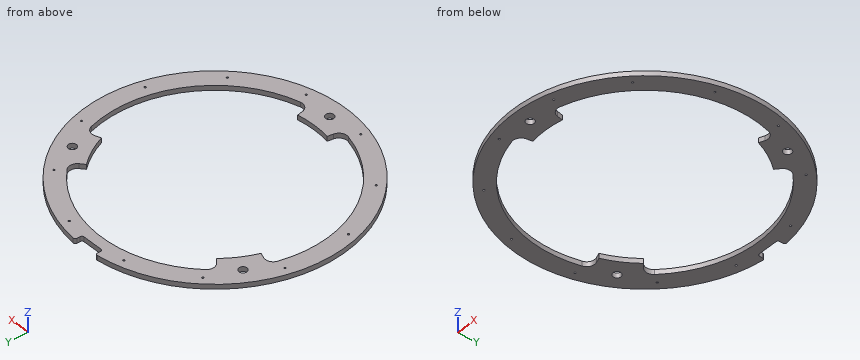
from build123d import *

# Parameters (mm, degrees)
SKETCH2_R                                      = 330
SKETCH2_R_2                                    = 250
BOSS_EXTRUDE1_DEPTH                            = 12
CUT_EXTRUDE1_DEPTH                             = 12
SKETCH4_R                                      = 10
CUT_EXTRUDE2_DEPTH                             = 12
SKETCH5_W                                      = 60
SKETCH5_H                                      = 60
CUT_EXTRUDE3_DEPTH                             = 12
FILLET1_R                                      = 5
CSK_FOR_M4_FLAT_HEAD_MACHINE_SCREW_D           = 4.5
CSK_FOR_M4_FLAT_HEAD_MACHINE_SCREW_CSINK_D     = 9.4
CSK_FOR_M4_FLAT_HEAD_MACHINE_SCREW_CSINK_ANGLE = 90


with BuildPart() as part:
    # Sketch2 → Boss-Extrude1 (new body)
    with BuildSketch(Plane.XY):
        Circle(SKETCH2_R)
        Circle(SKETCH2_R_2, mode=Mode.SUBTRACT)
    extrude(amount=BOSS_EXTRUDE1_DEPTH)

    # Sketch3 → Cut-Extrude1 (cut)
    with BuildSketch(Plane.XY.offset(12)):
        with BuildLine():
            Line((191.51111078, 160.696902422), (202.422805046, 169.852901056))
            ThreePointArc((202.422805046, 169.852901056), (209.542560602, 184.184300077), (203.874000238, 199.14917029))
            ThreePointArc((203.874000238, 199.14917029), (0, 285), (-203.874000238, 199.14917029))
            ThreePointArc((-203.874000238, 199.14917029), (-209.542560602, 184.184300077), (-202.422805046, 169.852901056))
            Line((-202.422805046, 169.852901056), (-191.51111078, 160.696902422))
            ThreePointArc((-191.51111078, 160.696902422), (0, 250), (191.51111078, 160.696902422))
        make_face()
        with BuildLine():
            Line((43.412044417, -246.201938253), (45.885524698, -260.229742003))
            ThreePointArc((45.885524698, -260.229742003), (54.737002544, -273.561330694), (70.531240495, -276.134648522))
            ThreePointArc((70.531240495, -276.134648522), (246.817240079, -142.5), (274.405240732, 76.985478232))
            ThreePointArc((274.405240732, 76.985478232), (264.279563146, 89.377030617), (248.308329744, 90.376840947))
            Line((248.308329744, 90.376840947), (234.923155196, 85.505035831))
            ThreePointArc((234.923155196, 85.505035831), (216.506350946, -125), (43.412044417, -246.201938253))
        make_face()
        with BuildLine():
            Line((-234.923155196, 85.505035831), (-248.308329744, 90.376840947))
            ThreePointArc((-248.308329744, 90.376840947), (-264.279563146, 89.377030617), (-274.405240732, 76.985478232))
            ThreePointArc((-274.405240732, 76.985478232), (-246.817240079, -142.5), (-70.531240495, -276.134648522))
            ThreePointArc((-70.531240495, -276.134648522), (-54.737002544, -273.561330694), (-45.885524698, -260.229742003))
            Line((-45.885524698, -260.229742003), (-43.412044417, -246.201938253))
            ThreePointArc((-43.412044417, -246.201938253), (-216.506350946, -125), (-234.923155196, 85.505035831))
        make_face()
    extrude(amount=-CUT_EXTRUDE1_DEPTH, mode=Mode.SUBTRACT)

    # Sketch4 → Cut-Extrude2 (cut)
    with BuildSketch(Plane.XY.offset(12)):
        with Locations((0, -290)):
            Circle(SKETCH4_R)
        with Locations((-251.147367097, 145)):
            Circle(SKETCH4_R)
        with Locations((251.147367097, 145)):
            Circle(SKETCH4_R)
    extrude(amount=-CUT_EXTRUDE2_DEPTH, mode=Mode.SUBTRACT)

    # Sketch5 → Cut-Extrude3 (cut)
    with BuildSketch(Plane.XY.offset(12)):
        with Locations((0, 340)):
            Rectangle(SKETCH5_W, SKETCH5_H)
    extrude(amount=-CUT_EXTRUDE3_DEPTH, mode=Mode.SUBTRACT)

    # Fillet1
    fillet1_edges = [part.edges().sort_by_distance(p)[0] for p in [
        (30, 328.633534503, 6),
        (-30, 328.633534503, 6),
        (-30, 310, 6),
        (30, 310, 6),
    ]]
    fillet(fillet1_edges, radius=FILLET1_R)

    # CSK for M4 Flat Head Machine Screw (through all)
    with Locations(Plane(origin=(0, 0, -24), x_dir=(1, 0, 0), z_dir=(0, 0, -1))):
        with Locations((80.233903982, 299.43700615), (219.203102168, 219.203102168), (299.43700615, 80.233903982), (299.43700615, -80.233903982), (219.203102168, -219.203102168), (80.233903982, -299.43700615), (-80.233903982, -299.43700615), (-219.203102168, -219.203102168), (-299.43700615, -80.233903982), (-299.43700615, 80.233903982), (-219.203102168, 219.203102168), (-80.233903982, 299.43700615), (0, 0)):
            CounterSinkHole(CSK_FOR_M4_FLAT_HEAD_MACHINE_SCREW_D / 2, CSK_FOR_M4_FLAT_HEAD_MACHINE_SCREW_CSINK_D / 2, counter_sink_angle=CSK_FOR_M4_FLAT_HEAD_MACHINE_SCREW_CSINK_ANGLE)


solid = part.part
The listing builds one solid part. Answer for the finished solid, in the listing's coordinates (mm). Round coordinates to 2 decimals unless told otherwise and drop trailing zeros. Order: outer loops, then holes, each group sorted by start corner. A loop starts at its lowest first (then second) coordinate and runs counter-clockwise, first axis right, second up. Notation, with made-up numbers: (62.5, 11.5) -> (117.5, 11.5) arc R20 ccw to (117.5, 47.5) -> close; hole circle Ø3 at (-16.75, 28.5). An arc over 180 degrees is marked (long way). Write each question's results on one line, items separated by ' | '. Start each with the question number.
Q1. Find section D-D (z = 3.5). Give the number of separate pieces and of enclosed holes in the cut face, then the cut area to 3 significant figures.
Q2. Find section B-B (y = 0). Determine the outline of the cut face in (x, z), then the cut area to 3 significant figures.
Q3. Straight lines are drawn through the part: probe 1 along Y at (x, z) = (-300.5, 11); probe 2 along X at (y, z) = (136.5, 11.25); probe 3 along X at (y, z) = (299, 4). For each, find the intervals that lie inside material, in ascending order. Write a range as from..to.
Q4. Find section A-A (x = 0). Determine the outline of the cut face in (y, z).
Q5. Find section C-C (y = 119.5). Determine the outline of the cut face in (x, z).
Q6. Each of these flat-tipped pins is pushed along its axis until it touches: pin 1 (1 mm diameter, centred on x = -202, z = 9, fed in from +Y); pin 2 (3 mm diameter, centred on y = -69, z = 10.5, fed in from -X); pin 3 (3.5 mm diameter, centred on x = -6.5, z = 3.5, fed in from +Y). Where does it stop, or does it pass through?
Worked answers:
1) separate pieces: 1 | enclosed holes: 16 | area: 95,000 mm2
2) outline: (-330, 0) -> (-285, 0) -> (-285, 12) -> (-330, 12) -> close; (285, 0) -> (330, 0) -> (330, 12) -> (285, 12) -> close | area: 1,080 mm2
3) probe 1: y = -136.38..-82.22, -78.25..78.25, 82.22..136.38 | probe 2: x = -300.45..-256.42, -245.88..-209.45, 209.45..245.88, 256.42..300.45 | probe 3: x = -139.64..-82.44, -78.03..78.03, 82.44..139.64
4) outline: (-330, 0) -> (-300, 0) -> (-300, 12) -> (-330, 12) -> close; (-280, 0) -> (-250, 0) -> (-250, 12) -> (-280, 12) -> close; (285, 0) -> (310, 0) -> (310, 12) -> (285, 12) -> close
5) outline: (-307.6, 0) -> (-219.59, 0) -> (-219.59, 12) -> (-307.6, 12) -> close; (219.59, 0) -> (307.6, 0) -> (307.6, 12) -> (219.59, 12) -> close
6) pin 1: stops at y = 261.34 | pin 2: stops at x = -323.02 | pin 3: stops at y = 310
